Design review of the part built by this model. Coordinates are the model's own, in mm. A direction names the side the tool comes from. Coordinates: 2 decimals unless noted, no trailing zeros. Write each loop counter-clockwise with the first axis right and the second up, starting at its lowest first coordinate (ties: lowest second). Pieces come first, ordered by that corner, then holes. Notation, with made-up numbers: (77, -36) - (106, -36) arc R14 cw to (106, -10) - close; hole circle Ø7 at (63.5, 5). An arc over 180 degrees is marked (long way). Answer as a JSON object with one key per item and string values.
```python
from build123d import *

# Parameters (mm, degrees)
RESSALTO_EXTRUS_O1_DEPTH = 15
ESBO_O2_R                = 2.5
CORTE_EXTRUS_O1_DEPTH    = 44.874821937
ESBO_O3_R                = 2.5
CORTE_EXTRUS_O2_DEPTH    = 6
FILETE1_R                = 1


with BuildPart() as part:
    # Esboço1 → Ressalto-extrusão1 (new body)
    with BuildSketch(Plane.XY):
        Polygon((0, 0), (0, 40), (10, 30), (10, 0), align=None)
    extrude(amount=RESSALTO_EXTRUS_O1_DEPTH)

    # Esboço2 → Corte-extrusão1 (cut, through all)
    with BuildSketch(Plane(origin=(10, 0, 0), x_dir=(0, 0, -1), z_dir=(1, 0, 0))):
        with Locations(Location((-6, 6, 0), (0, 0, 90))):
            Circle(ESBO_O2_R)
    extrude(amount=-CORTE_EXTRUS_O1_DEPTH, mode=Mode.SUBTRACT)

    # Esboço3 → Corte-extrusão2 (cut)
    with BuildSketch(Plane(origin=(0, 0, 0), x_dir=(-1, 0, 0), z_dir=(0, 0, -1))):
        with Locations((-2.5, 6)):
            Circle(ESBO_O3_R)
        with BuildLine():
            Line((0, 8.5), (-2.5, 8.5))
            ThreePointArc((-2.5, 8.5), (-0.732233047, 7.767766953), (0, 6))
            Line((0, 6), (0, 8.5))
        make_face()
        with BuildLine():
            Line((0, 3.5), (0, 6))
            ThreePointArc((0, 6), (-0.732233047, 4.232233047), (-2.5, 3.5))
            Line((-2.5, 3.5), (0, 3.5))
        make_face()
    extrude(amount=-CORTE_EXTRUS_O2_DEPTH, mode=Mode.SUBTRACT)

    # Filete1
    filete1_edges = [part.edges().sort_by_distance(p)[0] for p in [
        (10, 30, 7.5),
    ]]
    fillet(filete1_edges, radius=FILETE1_R)


solid = part.part
```
(1) To check wall thickness, follow line 1 (Z direction, x = 7, y = 6); line 2 (Y direction, x = 8.25, z = 6); line 3 (Z direction, x = 9.5, y = 8). State the ranges of each line that lie inside material, in increasing order. Write a range as from..to.
Solved:
{"line 1": "z = 0..3.5, 8.5..15", "line 2": "y = 0..3.5, 8.5..31.75", "line 3": "z = 0..4.5, 7.5..15"}
(2) Take a section at C-C, the plane z = 1.25. Write out the cut boundary in (x, y), and give its area (3 significant figures).
Solved:
{"outline": "(0, 0) - (10, 0) - (10, 29.59) arc R1 ccw to (9.71, 30.29) - (0, 40) - (0, 8.5) - (2.5, 8.5) arc R2.5 cw to (2.5, 3.5) - (0, 3.5) - close", "area": "328 mm^2"}
(3) Take a section at D-D, the plane x = 8.75. Write out the cut boundary in (y, z), and give its area (3 significant figures).
Solved:
{"outline": "(0, 0) - (31.25, 0) - (31.25, 15) - (0, 15) - close; hole circle Ø5 at (6, 6)", "area": "449 mm^2"}
(4) The part is to be moulded in two halves that separate along Y. For faces 1 (the face through (5, 16, 15)), 2 (the face through (1, 3.5, 3)), 3 (the face through (5, 35, 7)), say which applies: pulls with the +Y half, pulls with the -Y half, needs draft (parallel to the pull), parting line crosses it, or undercut.
Solved:
{"face 1": "needs draft", "face 2": "undercut", "face 3": "pulls with the +Y half"}
(5) Take a section at B-B, the plane y = 4. Write out the cut boundary in (x, z), and give its area (3 significant figures).
Solved:
{"outline": "(0, 7.5) - (10, 7.5) - (10, 15) - (0, 15) - close; (4, 0) - (10, 0) - (10, 4.5) - (4, 4.5) - close", "area": "102 mm^2"}
(6) For pin 1 (4 mm diameter, centred on x = 6, z = 4, fed in from +Y); pin 2 (1.5 mm diameter, centred on x = 5, z = 9.5, fed in from +Y); pin 3 (3 mm diameter, centred on x = 3.5, z = 7, fed in from +Y); pin 4 (4 mm diameter, centred on y = 6, z = 6, fed in from -X), all flat-tipped, find the tip position at first contact; note any pin that passes through.
Solved:
{"pin 1": "stops at y = 36", "pin 2": "stops at y = 35.75", "pin 3": "stops at y = 38", "pin 4": "passes through"}
(7) Take a section at A-A, the plane z = 8. Write out the cut boundary in (x, y), and give its area (3 significant figures).
Solved:
{"outline": "(0, 0) - (10, 0) - (10, 4.5) - (0, 4.5) - close; (0, 7.5) - (10, 7.5) - (10, 29.59) arc R1 ccw to (9.71, 30.29) - (0, 40) - close", "area": "320 mm^2"}
(8) Tool access review of faces 4 (the face through (5, 0, 7)), 5 (the face through (5, 6, 2)): name each direction out of +Z, -Z, +X, -X, +Y, -Y from which nothing blocks a thin tool from reaching the whole face with its end or side.
Solved:
{"face 4": "+Z, -Z, +X, -X, -Y", "face 5": "-Z, -X"}
